Work out the finished part from the listing and answer in its coordinate system (mm). Face numbers are marked on the shaded views. A direction names the side the tool comes from. Coordinates: 2 decimals unless noted, no trailing zeros. Write each loop counter-clockwise with the first axis right and the second up, starting at its lowest first coordinate (ties: lowest second). Pieces come first, ordered by that corner, then holes. Notation, with made-up numbers: (28, 71) - (87, 71) arc R15 cw to (87, 98) - close; hole circle Ø6 at (77.25, 9.25). An arc over 180 degrees is marked (long way). Use a Markdown table: item, result. Add a question column.
(1) Find the intervals of material crossed by line 1 (Y direction, x = -9.75, z = 0); line 2 (Z direction, x = -4.75, y = 0); line 3 (Y direction, x = 7, z = 24), in increasing order. Write a range as from..to.
(2) Given pin 1 Ø12 at (y, z) = (39.5, 26) entering from -X; pin 2 Ø3 at (y, z) = (12.5, -31) entering from -X; pin 3 Ø18.5 at (y, z) = (-23.5, -3) entering from +X, each flat-ended and moving along its own axis, determine where each tip first touches the part or whether it passes through.
(3) For a pull along Y with two mould halves and no side action, classify the marked faces 4 and 5 as released by +Y, released by -Y, zero draft, split by the parting line, or undercut.
(4) A tool of negligible diameter and unlimited length cuts with its end or side. For the marked faces 1, 2 and 3, from which of +Z, -Z, +X, -X, +Y, -Y can it reach the whole face along a straight path? Write none if from no direction.
(5) The part is cut by section A-A, the plane x = -10.5. Give the vertices of the cut face in (y, z), then the cut area to 3 significant figures.
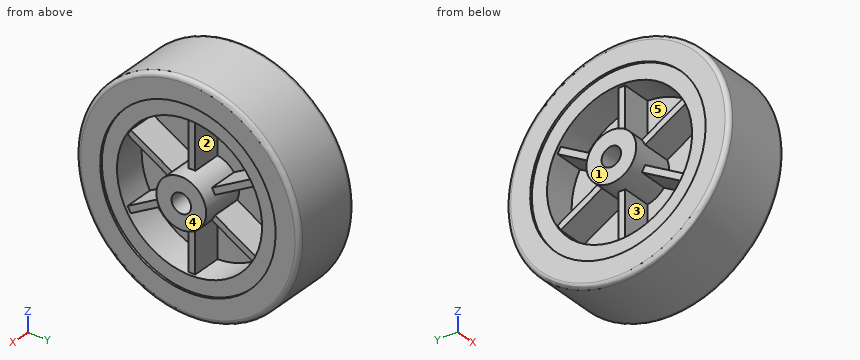
Solid Edge part; units mm, degrees
sketch "Sketch1" plane through (0, 0, 0) normal (0, -1, 0) x (1, 0, 0)
  line L0 (15.5, 40.5) -> (15.5, 33.5)
  line L1 (15.5, 33.5) -> (0.5, 33.5)
  line L2 (0.5, 33.5) -> (0.5, 11.5)
  line L3 (0.5, 11.5) -> (20.5, 11.5)
  line L4 (20.5, 11.5) -> (20.5, 4.5)
  line L5 (20.5, 4.5) -> (0, 4.5)
  line L6 (-20.5, 4.5) -> (0, 4.5)
  line L7 (-20.5, 11.5) -> (-20.5, 4.5)
  line L8 (-0.5, 11.5) -> (-20.5, 11.5)
  line L9 (-0.5, 33.5) -> (-0.5, 11.5)
  line L10 (-15.5, 33.5) -> (-0.5, 33.5)
  line L11 (-15.5, 40.5) -> (-15.5, 33.5)
  line L12 (-16.5, 40.5) -> (-15.5, 40.5)
  line L13 (-16.5, 51.5) -> (-16.5, 40.5)
  line L14 (0, 51.5) -> (-16.5, 51.5)
  line L15 (0, 51.5) -> (16.5, 51.5)
  line L16 (16.5, 51.5) -> (16.5, 40.5)
  line L17 (16.5, 40.5) -> (15.5, 40.5)
revolve "RevolvedProtrusion1" add sketch "Sketch1" angle 360 about axis through (0, 0, 0) along (1, 0, 0)
sketch "Sketch2" plane through (0, 0, 0) normal (1, 0, 0) x (0, 1, 0)
  line L0 (1.5, 10) -> (1.5, 35)
  line L1 (1.5, 35) -> (-1.5, 35)
  line L2 (-1.5, 35) -> (-1.5, 10)
  line L3 (-1.5, 10) -> (1.5, 10)
extrude "Protrusion1" add sketch "Sketch2" along normal mid plane 28
pattern_circular "Pattern1" count 6 over 360 about axis through (15.5, 0, 0) along (-1, 0, 0) of "Protrusion1"
fillet "arredondado_borracha" radius 2 2 edges at (16.5, 0, -51.5) (-16.5, 0, -51.5)
Model answer:
| question | item | result |
|---|---|---|
| 1 | line 1 | -51.5..-33.5, -11.5..-4.5, 4.5..11.5, 33.5..51.5 |
| 1 | line 2 | -51.5..-4.5, 4.5..51.5 |
| 1 | line 3 | -45.57..-23.37, -1.5..1.5, 23.37..45.57 |
| 2 | pin 1 | x = -16.5 |
| 2 | pin 2 | x = -15.5 |
| 2 | pin 3 | x = 14 |
| 3 | face 4 | zero draft |
| 3 | face 5 | undercut |
| 4 | face 1 | +Z, -Z, -X, +Y, -Y |
| 4 | face 2 | +X |
| 4 | face 3 | -X |
| 5 | outline | circle Ø103 at (0, 0); hole (-29.73, -15.43) - (-10.62, -4.4) arc R11.5 cw to (-10.62, 4.4) - (-29.73, 15.43) arc R33.5 ccw to start; hole (-28.23, -18.03) arc R33.5 ccw to (-1.5, -33.47) - (-1.5, -11.4) arc R11.5 cw to (-9.12, -7) - close; hole (-28.23, 18.03) - (-9.12, 7) arc R11.5 cw to (-1.5, 11.4) - (-1.5, 33.47) arc R33.5 ccw to start; hole circle Ø9 at (0, 0); hole (1.5, -33.47) arc R33.5 ccw to (28.23, -18.03) - (9.12, -7) arc R11.5 cw to (1.5, -11.4) - close; hole (1.5, 11.4) arc R11.5 cw to (9.12, 7) - (28.23, 18.03) arc R33.5 ccw to (1.5, 33.47) - close; hole (10.62, -4.4) - (29.73, -15.43) arc R33.5 ccw to (29.73, 15.43) - (10.62, 4.4) arc R11.5 cw to start |
| 5 | area | 5,550 mm^2 |
